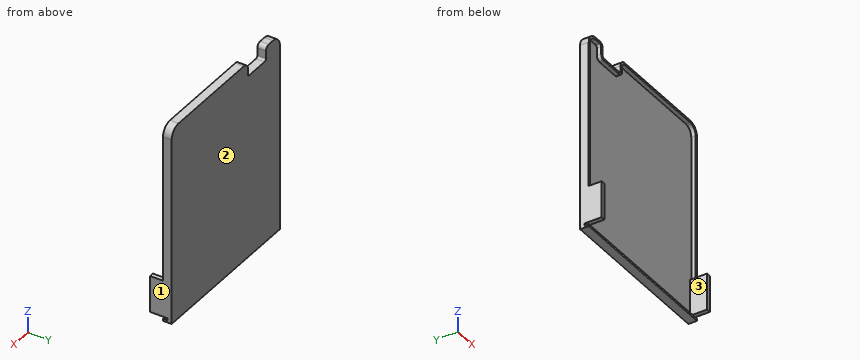
```python
from build123d import *

# Parameters (mm, degrees)
EXTRUDE_1_DEPTH = 2
EXTRUDE_START   = -4
SKETCH_2_W      = 78
SKETCH_2_H      = 1
EXTRUDE_2_DEPTH = 4
SKETCH_3_W      = 2
SKETCH_3_H      = 17.002857219
EXTRUDE_4_DEPTH = 10
SKETCH_5_W      = 1
SKETCH_5_H      = 1
EXTRUDE_6_DEPTH = 2


with BuildPart() as part:
    # Эскиз1 → Бобышка-Вытянуть1 (new body)
    with BuildSketch(Plane(origin=(0, 0, 0), x_dir=(1, 0, 0), z_dir=(0, 1, 0))):
        with BuildLine():
            Line((-39.421663854, 15.772857219), (-39.421663854, -47.227142781))
            ThreePointArc((-39.421663854, -47.227142781), (-38.250090979, -50.055569906), (-35.421663854, -51.227142781))
            Line((-35.421663854, -51.227142781), (-32.421663854, -51.227142781))
            ThreePointArc((-32.421663854, -51.227142781), (-31.714557073, -50.934249562), (-31.421663854, -50.227142781))
            Line((-31.421663854, -50.227142781), (-31.421663854, -46.727142781))
            ThreePointArc((-31.421663854, -46.727142781), (-30.835877417, -45.312929219), (-29.421663854, -44.727142781))
            Line((-29.421663854, -44.727142781), (-18.421663854, -44.727142781))
            ThreePointArc((-18.421663854, -44.727142781), (-17.007450292, -45.312929219), (-16.421663854, -46.727142781))
            Line((-16.421663854, -46.727142781), (-16.421663854, -49.227142781))
            ThreePointArc((-16.421663854, -49.227142781), (-15.835877417, -50.641356343), (-14.421663854, -51.227142781))
            Line((-14.421663854, -51.227142781), (21.578336146, -51.227142781))
            Line((21.578336146, -51.227142781), (32.578336146, -51.227142781))
            ThreePointArc((32.578336146, -51.227142781), (35.40676327, -50.055569906), (36.578336146, -47.227142781))
            Line((36.578336146, -47.227142781), (36.578336146, 15.772857219))
            Line((36.578336146, 15.772857219), (36.578336146, 38.772857219))
            Line((36.578336146, 38.772857219), (-39.421663854, 38.772857219))
            Line((-39.421663854, 38.772857219), (-39.421663854, 15.772857219))
        make_face()
    extrude(amount=EXTRUDE_1_DEPTH)

    # Эскиз2 → Бобышка-Вытянуть2 (add)
    with BuildSketch(Plane(origin=(0, 2, 0), x_dir=(1, 0, 0), z_dir=(0, 1, 0)).offset(EXTRUDE_START)):
        with BuildLine():
            Line((-35.421663854, -51.227142781), (-32.421663854, -51.227142781))
            ThreePointArc((-32.421663854, -51.227142781), (-31.714557073, -50.934249562), (-31.421663854, -50.227142781))
            Line((-31.421663854, -50.227142781), (-31.421663854, -46.727142781))
            ThreePointArc((-31.421663854, -46.727142781), (-30.835877417, -45.312929219), (-29.421663854, -44.727142781))
            Line((-29.421663854, -44.727142781), (-18.421663854, -44.727142781))
            ThreePointArc((-18.421663854, -44.727142781), (-17.007450292, -45.312929219), (-16.421663854, -46.727142781))
            Line((-16.421663854, -46.727142781), (-16.421663854, -49.227142781))
            ThreePointArc((-16.421663854, -49.227142781), (-15.835877417, -50.641356343), (-14.421663854, -51.227142781))
            Line((-14.421663854, -51.227142781), (32.578336146, -51.227142781))
            ThreePointArc((32.578336146, -51.227142781), (35.40676327, -50.055569906), (36.578336146, -47.227142781))
            Line((36.578336146, -47.227142781), (36.578336146, 15.772857219))
            Line((36.578336146, 15.772857219), (36.578336146, 21.77))
            Line((36.578336146, 21.77), (37.578336146, 21.77))
            Line((37.578336146, 21.77), (37.578336146, 15.772857219))
            Line((37.578336146, 15.772857219), (37.578336146, -47.227142781))
            ThreePointArc((37.578336146, -47.227142781), (36.113870052, -50.762676687), (32.578336146, -52.227142781))
            Line((32.578336146, -52.227142781), (-14.421663854, -52.227142781))
            ThreePointArc((-14.421663854, -52.227142781), (-16.542984198, -51.348463125), (-17.421663854, -49.227142781))
            Line((-17.421663854, -49.227142781), (-17.421663854, -46.727142781))
            ThreePointArc((-17.421663854, -46.727142781), (-17.714557073, -46.020036), (-18.421663854, -45.727142781))
            Line((-18.421663854, -45.727142781), (-29.421663854, -45.727142781))
            ThreePointArc((-29.421663854, -45.727142781), (-30.128770635, -46.020036), (-30.421663854, -46.727142781))
            Line((-30.421663854, -46.727142781), (-30.421663854, -50.227142781))
            ThreePointArc((-30.421663854, -50.227142781), (-31.007450292, -51.641356343), (-32.421663854, -52.227142781))
            Line((-32.421663854, -52.227142781), (-35.421663854, -52.227142781))
            ThreePointArc((-35.421663854, -52.227142781), (-38.95719776, -50.762676687), (-40.421663854, -47.227142781))
            Line((-40.421663854, -47.227142781), (-40.421663854, 15.772857219))
            Line((-40.421663854, 15.772857219), (-40.421663854, 21.77))
            Line((-40.421663854, 21.77), (-39.421663854, 21.77))
            Line((-39.421663854, 21.77), (-39.421663854, 15.772857219))
            Line((-39.421663854, 15.772857219), (-39.421663854, -47.227142781))
            ThreePointArc((-39.421663854, -47.227142781), (-38.250090979, -50.055569906), (-35.421663854, -51.227142781))
        make_face()
        with Locations((-1.421663854, 39.272857219)):
            Rectangle(SKETCH_2_W, SKETCH_2_H)
    extrude(amount=EXTRUDE_2_DEPTH)

    # Эскиз3 → Бобышка-Вытянуть4 (add)
    with BuildSketch(Plane(origin=(0, 2, 0), x_dir=(1, 0, 0), z_dir=(0, 1, 0))):
        with Locations((-39.421663854, 29.271428609)):
            Rectangle(SKETCH_3_W, SKETCH_3_H)
        with Locations((36.578336146, 29.271428609)):
            Rectangle(SKETCH_3_W, SKETCH_3_H)
    extrude(amount=-EXTRUDE_4_DEPTH)

    # Эскиз5 → Бобышка-Вытянуть6 (add)
    with BuildSketch(Plane(origin=(0, 2, 0), x_dir=(1, 0, 0), z_dir=(0, 1, 0))):
        with Locations((-39.921663854, 38.272857219)):
            Rectangle(SKETCH_5_W, SKETCH_5_H)
        with Locations((37.078336146, 38.272857219)):
            Rectangle(SKETCH_5_W, SKETCH_5_H)
    extrude(amount=-EXTRUDE_6_DEPTH)


solid = part.part
```
The model under review builds one solid part; all positions refer to its coordinate system, in mm. Face numbers are marked on the shaded views. Give positions to 0.01 mm unless a question says otherwise; leave off trailing zeros. Loops run counter-clockwise (first coordinate to the right, second up) from the corner with the lowest first, then second, coordinate; pieces in that order, holes last. Notation, with made-up numbers: (27.5, 77) -> (59.5, 77) arc R35 cw to (59.5, 113) -> close; hole circle Ø3 at (-12, -13.75). An arc over 180 degrees is marked (long way). Use CSV: the item, a comma, the result in double quotes.
1. Consider section A-A, the plane y = -4. Write out the cut boundary in (x, z), then the cut area to 3 significant figures.
Result:
outline,"(-40.42, -37.77) -> (-38.42, -37.77) -> (-38.42, -20.77) -> (-40.42, -20.77) -> close; (35.58, -37.77) -> (37.58, -37.77) -> (37.58, -20.77) -> (35.58, -20.77) -> close"
area,"68.0 mm²"
2. To check wall thickness, follow probe 1 along X at (y, z) = (-1, -19.5); probe 2 along Z at (x, y) = (-1, -1.5); probe 3 along Y at (x, z) = (8, -8). State the ranges of each line that lie inside material, in increasing order. Write a range as from..to.
Result:
probe 1,"x = -40.42..-39.42, 36.58..37.58"
probe 2,"z = -39.77..-38.77, 51.23..52.23"
probe 3,"y = 0..2"
3. For P1, Ø1, axis at x = 36.5, y = -6, coming from the -Z side; P2, Ø1, axis at x = -39.5, y = -5, coming from the +Z side; P3, Ø2, axis at x = 16.5, z = -23.5, coming from the -Y side, all flat-tipped, find the tip position at first contact; note any pin that passes through.
Result:
P1,"stops at z = -37.77"
P2,"stops at z = -20.77"
P3,"stops at y = 0"
4. Consider section B-B, the plane z = 35. Write out the cut boundary in (x, y), then the cut area to 3 significant figures.
Result:
outline,"(-40.42, -2) -> (-39.42, -2) -> (-39.42, 0) -> (36.58, 0) -> (36.58, -2) -> (37.58, -2) -> (37.58, 2) -> (-40.42, 2) -> close"
area,"160 mm²"
5. Consider section C-C, the plane x = 13. Write out the cut boundary in (y, z).
Result:
outline,"(-2, -39.77) -> (2, -39.77) -> (2, 52.23) -> (-2, 52.23) -> (-2, 51.23) -> (0, 51.23) -> (0, -38.77) -> (-2, -38.77) -> close"
6. The part is to be moulded in two halves that separate along X. For the marked faces 1, 2 and 3, say which applies: +X half, -X half, draft (parallel to the pull), parting line (faces both ways), or undercut.
Result:
face 1,"+X half"
face 2,"draft"
face 3,"undercut"
